Could you check a few things on this drawing? It's one solid part, dimensions in mm from its lowest x, y, z. A direction names the side the tool comes from. Coordinates: 2 decimals unless noted, no trailing zeros. Order: outer loops, then holes, each group sorted by start corner. A loop starts at its lowest first (then second) coordinate and runs counter-clockwise, first axis right, second up. Notation, with made-up numbers: (57.25, -39) - (103.25, -39) arc R22 ccw to (103.25, 0) - close; hole circle Ø8 at (-8.75, -23.75). An arc over 180 degrees is marked (long way). Answer in a Markdown table with one row per item. Add a question column.
Item 1: On a 3-axis mill with a long thin cutter (end or side, diameter ignored), from which of +Z, -Z, +X, -X, +Y, -Y can I reach the whole of each face in a straight line? I mean the marked faces 1, 2 and 3. Say none if no direction works.
Item 2: I want a section at B-B (y = 86). Please give me the cut outline in (x, z).
Item 3: I want a section at C-C (z = 15). Please give me the cut outline in (x, y).
Item 4: Thinking about a two-plate mould opening in X: for the marked faces 4, 5, 6 and 7, which applies, +X half, -X half, draft (parallel to the pull), parting line (faces both ways), or undercut?
Item 5: I want a section at A-A (z = 5). Please give me the cut outline in (x, y).
Item 6: I want a section at D-D (x = 10.5). Please give me the cut outline in (y, z), plus the area to 3 significant figures.
Item 7: Will these pins go through, and if not, where does the flat tip stop? pin 1 Ø12 at (y, z) = (52.5, 6) entering from +X; pin 2 Ø1.5 at (x, z) = (8.5, 7.5) entering from +Y; pin 3 Ø8 at (x, z) = (9, 17.5) entering from +Y; pin 4 Ø5 at (x, y) = (7.5, 39.5) entering from -Z.
Item 8: If I drill on line 1 along Y through (x, z) = (14.3, 15); line 2 along X through (y, z) = (3.9, 5); line 3 along Z through (x, y) = (14.7, 86), over which ranges is the centre line in solid material (lowest first)? Write a range as from..to.
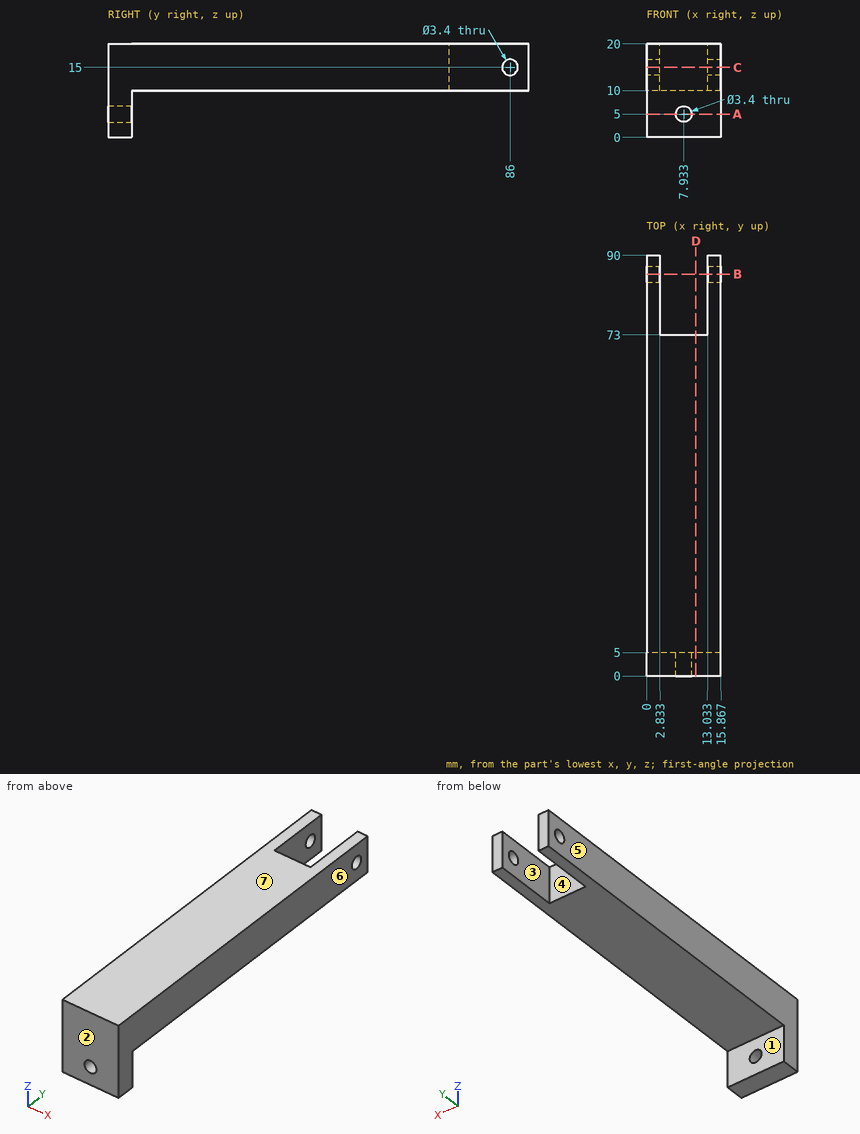
Values follow:
| question | item | result |
|---|---|---|
| 1 | face 1 | -Z, +X, -X, +Y |
| 1 | face 2 | +Z, -Z, +X, -X, -Y |
| 1 | face 3 | +Z, -Z, +Y |
| 2 | outline | (0, 10) - (2.83, 10) - (2.83, 13.3) - (0, 13.3) - close; (0, 16.7) - (2.83, 16.7) - (2.83, 20) - (0, 20) - close; (13.03, 10) - (15.87, 10) - (15.87, 13.3) - (13.03, 13.3) - close; (13.03, 16.7) - (15.87, 16.7) - (15.87, 20) - (13.03, 20) - close |
| 3 | outline | (0, 0) - (15.87, 0) - (15.87, 84.3) - (13.03, 84.3) - (13.03, 73) - (2.83, 73) - (2.83, 84.3) - (0, 84.3) - close; (0, 87.7) - (2.83, 87.7) - (2.83, 90) - (0, 90) - close; (13.03, 87.7) - (15.87, 87.7) - (15.87, 90) - (13.03, 90) - close |
| 4 | face 4 | undercut |
| 4 | face 5 | -X half |
| 4 | face 6 | +X half |
| 4 | face 7 | draft |
| 5 | outline | (0, 0) - (6.23, 0) - (6.23, 5) - (0, 5) - close; (9.63, 0) - (15.87, 0) - (15.87, 5) - (9.63, 5) - close |
| 6 | outline | (0, 0) - (5, 0) - (5, 10) - (73, 10) - (73, 20) - (0, 20) - close |
| 6 | area | 780 mm^2 |
| 7 | pin 1 | stops at x = 15.87 |
| 7 | pin 2 | stops at y = 5 |
| 7 | pin 3 | stops at y = 73 |
| 7 | pin 4 | stops at z = 10 |
| 8 | line 1 | y = 0..84.3, 87.7..90 |
| 8 | line 2 | x = 0..6.23, 9.63..15.87 |
| 8 | line 3 | z = 10..13.3, 16.7..20 |
